Can you work these out from the drawing? Everything is in mm from the part's minimum corner. A direction names the side the tool comes from. Give positions to 0.01 mm unless a question says otherwise; leave off trailing zeros. Loops run counter-clockwise (first coordinate to the right, second up) from the corner with the lowest first, then second, coordinate; pieces in that order, holes last. Notation, with made-up numbers: (62.25, -8.75) - (67.25, -8.75) arc R26 cw to (67.25, 24.25) - close; hole circle Ø2 at (66, 89). An arc over 180 degrees is marked (long way). One line per item, written item: value. Start each with the question number.
Q1. I want a section at A-A (y = 41.05). Please give me the cut outline in (x, z), then the cut area to 3 significant figures.
Q2. If I drill on line 1 (Z direction, x = 2.3, y = 6); line 2 (X direction, y = 14.5, z = 22); line 3 (X direction, y = 15.5, z = 44), over which ranges is the centre line in solid material (lowest first)? Write a range as from..to.
Q3. If we mould it in two halves opening along X, with no side actions, what happens to the marked faces 1, 2 and 3? For each: released by +X, released by -X, zero draft, split by the parting line, or undercut.
Q4. I want a section at C-C (y = 6). Please give me the cut outline in (x, z).
Q5. I want a section at D-D (x = 2). Please give me the cut outline in (y, z).
Q6. I want a section at B-B (x = 11.75). Please give me the cut outline in (y, z).
Q7. For the marked faces 4, 5, 6 and 7, which set-ups out of +Z, -Z, +X, -X, +Y, -Y let a thin tool reach every point of the face, with its end or its side?
Q8. I'm going to push flat-ended pins straight in: P1, Ø3.5, axis at y = 43, z = 36, coming from the +X side; P2, Ø8, axis at x = 5, y = 20, coming from the -Z side; P3, Ø7.5, axis at x = 17.5, z = 38, coming from the +Y side; P4, Ø9.5, axis at x = 13.5, z = 13.5, coming from the -Y side. Where does each tip first touch, or does it pass through?
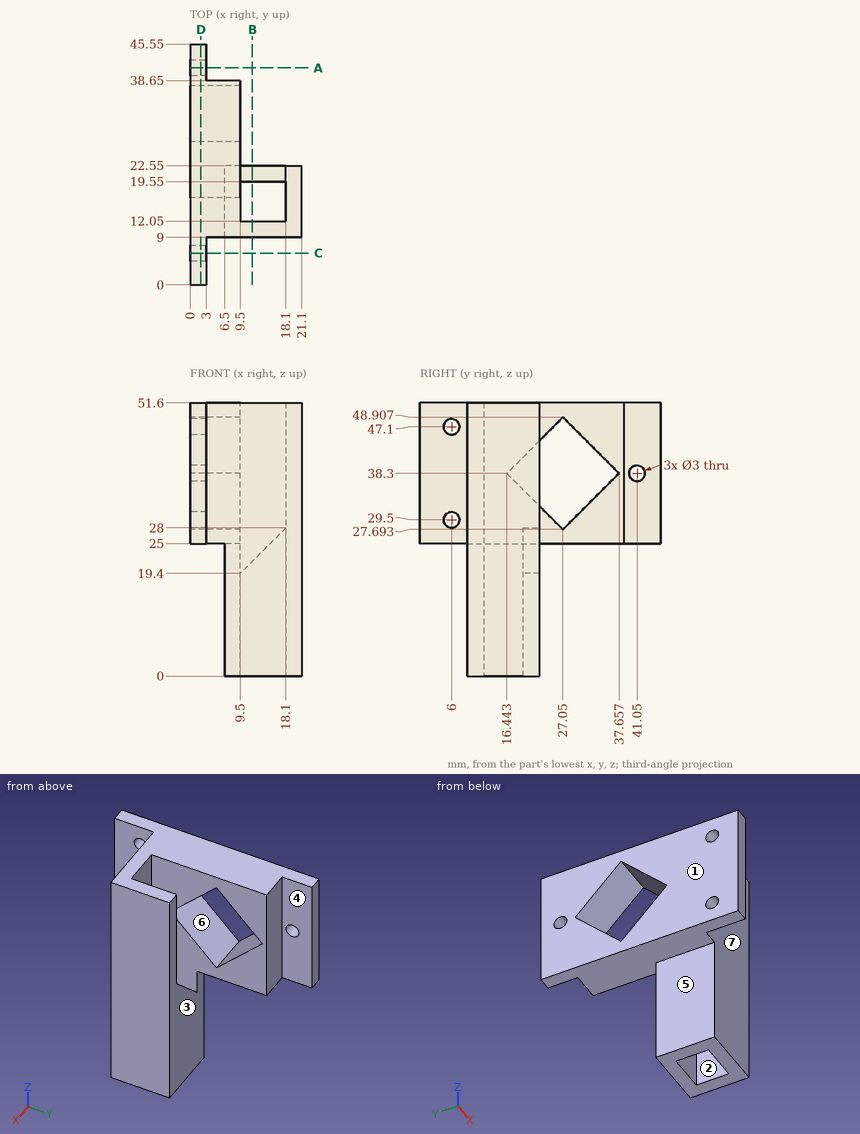
Worked answers:
1. outline: (0, 25) - (3, 25) - (3, 36.8) - (0, 36.8) - close; (0, 39.8) - (3, 39.8) - (3, 51.6) - (0, 51.6) - close
1. area: 70.8 mm²
2. line 1: z = 25..28, 31..45.6, 48.6..51.6
2. line 2: x = 6.5..9.5, 18.1..21.1
2. line 3: x = 0..9.5, 18.1..21.1
3. face 1: released by -X
3. face 2: undercut
3. face 3: zero draft
4. outline: (0, 25) - (3, 25) - (3, 28) - (0, 28) - close; (0, 31) - (3, 31) - (3, 45.6) - (0, 45.6) - close; (0, 48.6) - (3, 48.6) - (3, 51.6) - (0, 51.6) - close
5. outline: (0, 25) - (45.55, 25) - (45.55, 51.6) - (0, 51.6) - close; hole circle Ø3 at (6, 29.5); hole circle Ø3 at (6, 47.1); hole (16.44, 38.3) - (27.05, 27.69) - (37.66, 38.3) - (27.05, 48.91) - close; hole circle Ø3 at (41.05, 38.3)
6. outline: (9, 0) - (12.05, 0) - (12.05, 51.6) - (9, 51.6) - close; (19.55, 0) - (22.55, 0) - (22.55, 21.65) - (19.55, 21.65) - close
7. face 4: +Z, -Z, +X, +Y
7. face 5: -Z, -X, +Y, -Y
7. face 6: -X
7. face 7: +Z, -Z, +X, -Y
8. P1: stops at x = 3
8. P2: stops at z = 0
8. P3: stops at y = 22.55
8. P4: stops at y = 9
